Print and shaded views of the part. All mm, measured from the part's lowest x, y and z. Round coordinates to 2 decimals unless told otherwise and drop trailing zeros. Write each loop counter-clockwise with the first axis right and the second up, starting at its lowest first coordinate (ties: lowest second). Pieces come first, ordered by that corner, then holes. Notation, with made-up numbers: (37, 29) - (56, 29) arc R29 cw to (56, 66) - close; hole circle Ø5 at (-6.75, 13.25). An arc over 180 degrees is marked (long way). One line per item, written item: value.
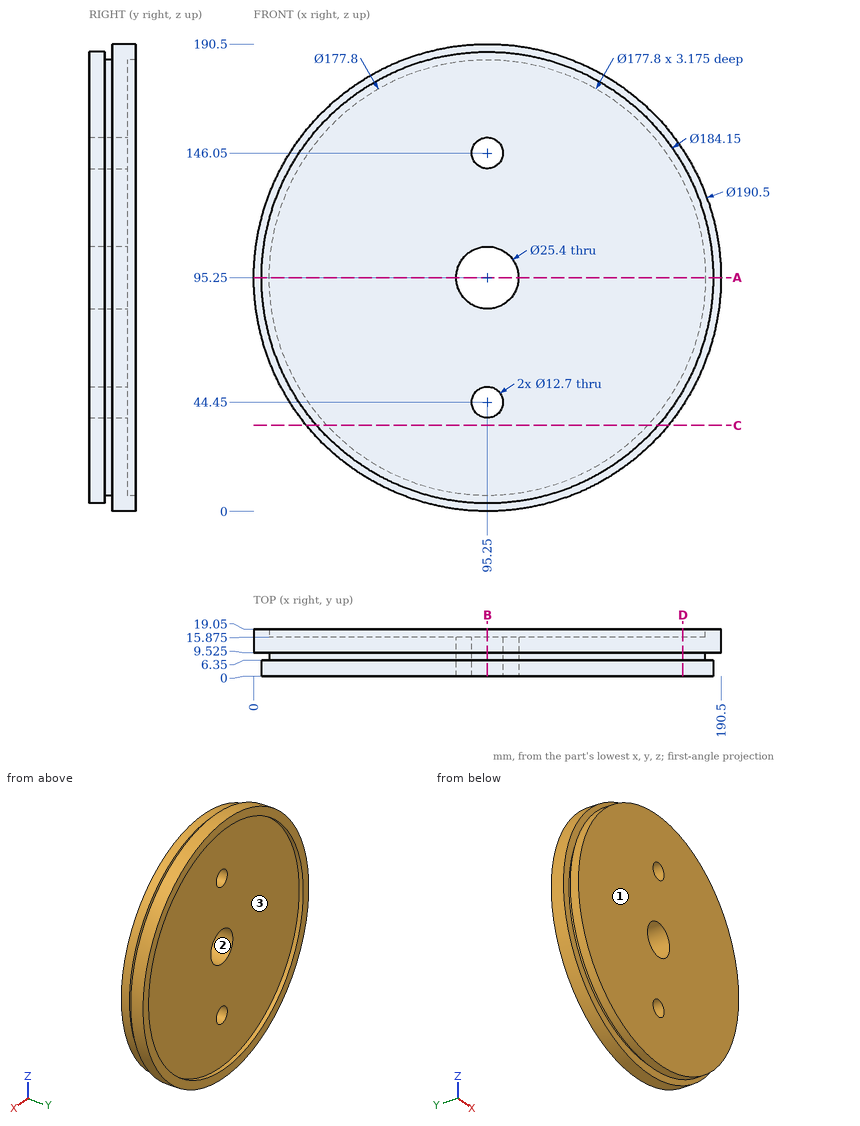
1. Band-saw the part on A-A on z = 95.25. Write the cut outline in (x, y) (3 decimals), plus the area to 3 significant figures.
Report:
outline: (0, 9.525) - (6.35, 9.525) - (6.35, 6.35) - (3.175, 6.35) - (3.175, 0) - (82.55, 0) - (82.55, 15.875) - (6.35, 15.875) - (6.35, 19.05) - (0, 19.05) - close; (107.95, 0) - (187.325, 0) - (187.325, 6.35) - (184.15, 6.35) - (184.15, 9.525) - (190.5, 9.525) - (190.5, 19.05) - (184.15, 19.05) - (184.15, 15.875) - (107.95, 15.875) - close
area: 2,580 mm²
2. Wall check: probe 1 along Z at (x, y) = (95.25, 6.5); probe 2 along Z at (x, y) = (95.25, 12.5); probe 3 along Z at (x, y) = (95.25, 17.9). Give the ranges that are in metal, low to high. Write a range as [from, to].
Report:
probe 1: [6.35, 38.1], [50.8, 82.55], [107.95, 139.7], [152.4, 184.15]
probe 2: [0, 38.1], [50.8, 82.55], [107.95, 139.7], [152.4, 190.5]
probe 3: [0, 6.35], [184.15, 190.5]
3. Band-saw the part on B-B on x = 95.25. Write the cut outline in (y, z) (3 decimals), plus the area to 3 significant figures.
Report:
outline: (0, 3.175) - (6.35, 3.175) - (6.35, 6.35) - (9.525, 6.35) - (9.525, 0) - (19.05, 0) - (19.05, 6.35) - (15.875, 6.35) - (15.875, 38.1) - (0, 38.1) - close; (0, 50.8) - (15.875, 50.8) - (15.875, 82.55) - (0, 82.55) - close; (0, 107.95) - (15.875, 107.95) - (15.875, 139.7) - (0, 139.7) - close; (0, 152.4) - (15.875, 152.4) - (15.875, 184.15) - (19.05, 184.15) - (19.05, 190.5) - (9.525, 190.5) - (9.525, 184.15) - (6.35, 184.15) - (6.35, 187.325) - (0, 187.325) - close
area: 2,180 mm²
4. Band-saw the part on D-D on x = 175. Write the cut outline in (y, z) (3 decimals), plus the area to 3 significant figures.
Report:
outline: (0, 49.231) - (6.35, 49.231) - (6.35, 55.967) - (9.525, 55.967) - (9.525, 43.168) - (19.05, 43.168) - (19.05, 55.967) - (15.875, 55.967) - (15.875, 134.533) - (19.05, 134.533) - (19.05, 147.332) - (9.525, 147.332) - (9.525, 134.533) - (6.35, 134.533) - (6.35, 141.269) - (0, 141.269) - close
area: 1,580 mm²
5. Band-saw the part on C-C on z = 35. Write the cut outline in (x, y) (3 decimals), plus the area to 3 significant figures.
Report:
outline: (21.477, 9.525) - (29.881, 9.525) - (29.881, 6.35) - (25.624, 6.35) - (25.624, 0) - (164.876, 0) - (164.876, 6.35) - (160.619, 6.35) - (160.619, 9.525) - (169.023, 9.525) - (169.023, 19.05) - (160.619, 19.05) - (160.619, 15.875) - (29.881, 15.875) - (29.881, 19.05) - (21.477, 19.05) - close
area: 2,290 mm²
6. Mould opens along X. For the marked faces 1, 2 and 3 say: released by +X, released by -X, zero draft, split by the parting line, or undercut.
Report:
face 1: zero draft
face 2: undercut
face 3: undercut
7. Drop flat-ended pins along their axis: pin 1 (8 mm diameter, centred on y = 11.5, z = 52, fed in from +X); pin 2 (5 mm diameter, centred on y = 6, z = 149, fed in from -X); pin 3 (3 mm diameter, centred on x = 80, y = 13, fed in from +Z); pin 4 (10 mm diameter, centred on x = 95.25, z = 146.05, fed in from -Y). Give the stop position or say it passes through.
Report:
pin 1: x = 182.04
pin 2: x = 18.76
pin 3: z = 189.5
pin 4: through
